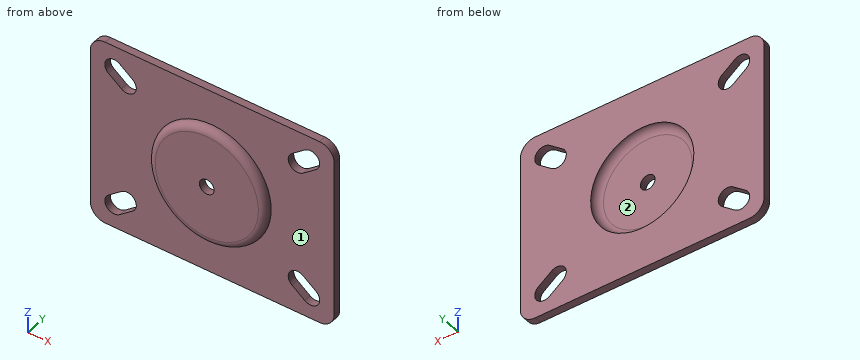
```python
from build123d import *

# Parameters (mm, degrees)
SKETCH12_W          = 105
SKETCH12_H          = 80
BOSS_EXTRUDE6_DEPTH = 3.175
SKETCH15_R          = 25.4
BOSS_EXTRUDE7_DEPTH = 6.35
SKETCH16_R          = 22.225
CUT_EXTRUDE3_DEPTH  = 3.175
CUT_EXTRUDE2_REACH  = 68.307
SKETCH14_R          = 3.175
FILLET6_R           = 6.35
FILLET7_R           = 3.175


with BuildPart() as part:
    # Sketch12 → Boss-Extrude6 (new body)
    with BuildSketch(Plane(origin=(0, 0, 0), x_dir=(-1, 0, 0), z_dir=(0, 1, 0))):
        Rectangle(SKETCH12_W, SKETCH12_H)
    extrude(amount=BOSS_EXTRUDE6_DEPTH)

    # Sketch15 → Boss-Extrude7 (add)
    with BuildSketch(Plane(origin=(0, 3.175, 0), x_dir=(1, 0, 0), z_dir=(0, 1, 0))):
        with Locations(Location((0, 0, 0), (0, 0, 270))):
            Circle(SKETCH15_R)
    extrude(amount=-BOSS_EXTRUDE7_DEPTH)

    # Sketch16 → Cut-Extrude3 (cut)
    with BuildSketch(Plane(origin=(0, 3.175, 0), x_dir=(1, 0, 0), z_dir=(0, 1, 0))):
        with Locations(Location((0, 0, 0), (0, 0, 270))):
            Circle(SKETCH16_R)
    extrude(amount=-CUT_EXTRUDE3_DEPTH, mode=Mode.SUBTRACT)

    # Sketch14 → Cut-Extrude2 (cut, up to next)
    with BuildSketch(Plane(origin=(0, 3.175, 0), x_dir=(-1, 0, 0), z_dir=(0, 1, 0)), mode=Mode.PRIVATE) as cut_extrude2_sk1:
        with Locations(Location((0, 0, 0), (0, 0, 90))):
            Circle(SKETCH14_R)
    cut_extrude2_tool1 = extrude(cut_extrude2_sk1.sketch, amount=-CUT_EXTRUDE2_REACH, mode=Mode.PRIVATE) & part.part
    # Sketch14 → Cut-Extrude2 (cut, up to next)
    with BuildSketch(Plane(origin=(0, 3.175, 0), x_dir=(-1, 0, 0), z_dir=(0, 1, 0)), mode=Mode.PRIVATE) as cut_extrude2_sk2:
        with BuildLine():
            Line((44.708183881, 26.939424373), (39.140161841, 22.697121866))
            ThreePointArc((39.140161841, 22.697121866), (33.5342621, 23.454675886), (34.291816119, 29.060575627))
            Line((34.291816119, 29.060575627), (39.859838159, 33.302878134))
            ThreePointArc((39.859838159, 33.302878134), (45.4657379, 32.545324114), (44.708183881, 26.939424373))
        make_face()
    cut_extrude2_tool2 = extrude(cut_extrude2_sk2.sketch, amount=-CUT_EXTRUDE2_REACH, mode=Mode.PRIVATE) & part.part
    # Sketch14 → Cut-Extrude2 (cut, up to next)
    with BuildSketch(Plane(origin=(0, 3.175, 0), x_dir=(-1, 0, 0), z_dir=(0, 1, 0)), mode=Mode.PRIVATE) as cut_extrude2_sk3:
        with BuildLine():
            Line((-44.708183881, 26.939424373), (-39.140161841, 22.697121866))
            ThreePointArc((-39.140161841, 22.697121866), (-33.5342621, 23.454675886), (-34.291816119, 29.060575627))
            Line((-34.291816119, 29.060575627), (-39.859838159, 33.302878134))
            ThreePointArc((-39.859838159, 33.302878134), (-45.4657379, 32.545324114), (-44.708183881, 26.939424373))
        make_face()
    cut_extrude2_tool3 = extrude(cut_extrude2_sk3.sketch, amount=-CUT_EXTRUDE2_REACH, mode=Mode.PRIVATE) & part.part
    # Sketch14 → Cut-Extrude2 (cut, up to next)
    with BuildSketch(Plane(origin=(0, 3.175, 0), x_dir=(-1, 0, 0), z_dir=(0, 1, 0)), mode=Mode.PRIVATE) as cut_extrude2_sk4:
        with BuildLine():
            Line((-44.708183881, -26.939424373), (-39.140161841, -22.697121866))
            ThreePointArc((-39.140161841, -22.697121866), (-33.5342621, -23.454675886), (-34.291816119, -29.060575627))
            Line((-34.291816119, -29.060575627), (-39.859838159, -33.302878134))
            ThreePointArc((-39.859838159, -33.302878134), (-45.4657379, -32.545324114), (-44.708183881, -26.939424373))
        make_face()
    cut_extrude2_tool4 = extrude(cut_extrude2_sk4.sketch, amount=-CUT_EXTRUDE2_REACH, mode=Mode.PRIVATE) & part.part
    # Sketch14 → Cut-Extrude2 (cut, up to next)
    with BuildSketch(Plane(origin=(0, 3.175, 0), x_dir=(-1, 0, 0), z_dir=(0, 1, 0)), mode=Mode.PRIVATE) as cut_extrude2_sk5:
        with BuildLine():
            Line((44.708183881, -26.939424373), (39.140161841, -22.697121866))
            ThreePointArc((39.140161841, -22.697121866), (33.5342621, -23.454675886), (34.291816119, -29.060575627))
            Line((34.291816119, -29.060575627), (39.859838159, -33.302878134))
            ThreePointArc((39.859838159, -33.302878134), (45.4657379, -32.545324114), (44.708183881, -26.939424373))
        make_face()
    cut_extrude2_tool5 = extrude(cut_extrude2_sk5.sketch, amount=-CUT_EXTRUDE2_REACH, mode=Mode.PRIVATE) & part.part
    add(cut_extrude2_tool1.solids().sort_by_distance((0, 3.175, 0))[0], mode=Mode.SUBTRACT)
    add(cut_extrude2_tool2.solids().sort_by_distance((-39.5, 3.175, 28))[0], mode=Mode.SUBTRACT)
    add(cut_extrude2_tool3.solids().sort_by_distance((39.5, 3.175, 28))[0], mode=Mode.SUBTRACT)
    add(cut_extrude2_tool4.solids().sort_by_distance((39.5, 3.175, -28))[0], mode=Mode.SUBTRACT)
    add(cut_extrude2_tool5.solids().sort_by_distance((-39.5, 3.175, -28))[0], mode=Mode.SUBTRACT)

    # Fillet6
    fillet6_edges = [part.edges().sort_by_distance(p)[0] for p in [
        (52.5, 1.5875, 40),
        (-52.5, 1.5875, 40),
        (-52.5, 1.5875, -40),
        (52.5, 1.5875, -40),
    ]]
    fillet(fillet6_edges, radius=FILLET6_R)

    # Fillet7
    fillet7_edges = [part.edges().sort_by_distance(p)[0] for p in [
        (0, -3.175, -25.4),
        (0, 0, -22.225),
    ]]
    fillet(fillet7_edges, radius=FILLET7_R - 0.0001)  # a hair under: the kernel refuses the full size


solid = part.part
```
Verification items for the finished model (mm, model axes). Face numbers are marked on the shaded views. Coordinates: 2 decimals unless noted, no trailing zeros. Write each loop counter-clockwise with the first axis right and the second up, starting at its lowest first coordinate (ties: lowest second). Pieces come first, ordered by that corner, then holes. Notation, with made-up numbers: (34.5, 81) - (73.5, 81) arc R13 ccw to (73.5, 85) - close; hole circle Ø5 at (69.25, -18.5). An arc over 180 degrees is marked (long way). Write item = value, one per line.
Q1. Cross-section at D-D (y = 1.75). Enter the section's corners in (x, z).
Answer:
outline = (-52.5, -33.65) arc R6.35 ccw to (-46.15, -40) - (46.15, -40) arc R6.35 ccw to (52.5, -33.65) - (52.5, 33.65) arc R6.35 ccw to (46.15, 40) - (-46.15, 40) arc R6.35 ccw to (-52.5, 33.65) - close; hole (-44.71, -26.94) arc R4 ccw to (-39.86, -33.3) - (-34.29, -29.06) arc R4 ccw to (-39.14, -22.7) - close; hole (-44.71, 26.94) - (-39.14, 22.7) arc R4 ccw to (-34.29, 29.06) - (-39.86, 33.3) arc R4 ccw to start; hole circle Ø43.77 at (0, 0); hole (34.29, -29.06) - (39.86, -33.3) arc R4 ccw to (44.71, -26.94) - (39.14, -22.7) arc R4 ccw to start; hole (34.29, 29.06) arc R4 ccw to (39.14, 22.7) - (44.71, 26.94) arc R4 ccw to (39.86, 33.3) - close
Q2. Material ranges on L1, parallel to X at y = 0.5, z = -25.5; L2, parallel to X at y = 1.75, z = 0.5; L3, parallel to Z at x = 47.5, y = 2, recorded low to high. Write a range as from..to.
Answer:
L1 = -52.5..-42.82, -32.73..32.73, 42.82..52.5
L2 = -52.5..-21.88, 21.88..52.5
L3 = -39.85..39.85
Q3. Mould release check, pull along Z, two halves, no side actions. Record for the marked faces 1 and 2: released by +Z, released by -Z, zero draft, split by the parting line, or undercut.
Answer:
face_1 = zero draft
face_2 = undercut
Q4. Cross-section at C-C (z = 31). Enter the section's corners in (x, y) (3 decimals).
Answer:
outline = (-52.5, 0) - (-46.186, 0) - (-46.186, 3.175) - (-52.5, 3.175) - close; (-36.837, 0) - (36.837, 0) - (36.837, 3.175) - (-36.837, 3.175) - close; (46.186, 0) - (52.5, 0) - (52.5, 3.175) - (46.186, 3.175) - close
Q5. Go/stop test with flat-tipped pins: pin 1 Ø5 at (x, z) = (0, 0) entering from +Y; pin 2 Ø5 at (x, z) = (-35.5, -24.5) entering from -Y. Record where each tip stops, or that it passes through.
Answer:
pin_1 = through
pin_2 = 0
